Geometry: final body of the model. Coordinates: model frame, mm. A direction names the side the tool comes from. Give positions to 0.01 mm unless a question says otherwise; leave off trailing zeros. Loops run counter-clockwise (first coordinate to the right, second up) from the corner with the lowest first, then second, coordinate; pieces in that order, holes last.
1. First-contact query: P1, Ø1.5, axis at x = -27.5, z = 3.5, coming from the -Y side. Flat tip, straight axial feed; report the tip coordinate or a pass-through.
2. Section A-A, the plane y = 13. Output: boundary loops of the cut face in (x, z), then the cut area to 3 significant figures.
3. Access query for faces 5 (the face through (-29.15, 14.93, -0.92)), 6 (the face through (0.49, -1.745, -5.361)). Directions: +Z, -Z, +X, -X, +Y, -Y. A direction counts if a zero-diameter tool reaches every point of the face in a straight line with its end or side. Return the directions, or none.
4. Section D-D, the plane y = -0.75. Output: boundary loops of the cut face in (x, z).
5. Section C-C, the plane z = -6. Output: boundary loops of the cut face in (x, y), then the cut area to 3 significant figures.
6. Material intervals for line 1 along X through (y, z) = (6.25, -1); line 2 along X through (y, z) = (18, 0); line 3 along Z through (x, y) = (26, 15), sorted ascending.
7. Draft query along X for faces 1 (the face through (-35, 8, 0)), 2 (the face through (0, 12, 7.5)), 3 (the face through (35, 8, 0)), 4 (the face through (-29.063, 4.93, -0.902)). Return one class per face: +X half, -X half, draft (parallel to the pull), parting line (faces both ways), or undercut.
from build123d import *
from OCP.BRepFilletAPI import BRepFilletAPI_MakeChamfer

# Parameters (mm, degrees)
SKETCH1_W           = 70
SKETCH1_H           = 15
SKETCH1_R           = 4.25
BOSS_EXTRUDE1_DEPTH = 20
SKETCH2_W           = 70
SKETCH2_H           = 15
BOSS_EXTRUDE2_DEPTH = 4
FILLET1_R           = 7.5
CHAMFER1_SIZE       = 10
CHAMFER1_SIZE2      = 0.174550649


with BuildPart() as part:
    # Sketch1 → Boss-Extrude1 (new body)
    with BuildSketch(Plane(origin=(0, 0, 0), x_dir=(1, 0, 0), z_dir=(0, 1, 0))):
        Rectangle(SKETCH1_W, SKETCH1_H)
        with Locations(Location((-25, 0, 0), (0, 0, 270))):
            Circle(SKETCH1_R, mode=Mode.SUBTRACT)
        with Locations(Location((25, 0, 0), (0, 0, 270))):
            Circle(SKETCH1_R, mode=Mode.SUBTRACT)
    extrude(amount=BOSS_EXTRUDE1_DEPTH)

    # Sketch2 → Boss-Extrude2 (add)
    with BuildSketch(Plane.XZ):
        Rectangle(SKETCH2_W, SKETCH2_H)
    extrude(amount=BOSS_EXTRUDE2_DEPTH)

    # Fillet1
    fillet1_edges = [part.edges().sort_by_distance(p)[0] for p in [
        (0, -4, 7.5),
        (0, -4, -7.5),
    ]]
    fillet(fillet1_edges, radius=FILLET1_R - 0.0001)  # a hair under: the kernel refuses the full size

    # Chamfer1: one chamfer whose edges measure the first distance from different faces: ONE call of the kernel's chamfer builder (chamfer() names one face for all edges)
    chamfer1_edges_1 = [part.edges().sort_by_distance(p)[0] for p in [
        (-25, 0, -4.25),
    ]]
    chamfer1_side_1 = [part.faces().sort_by_distance(p)[0] for p in [
        (-25, 10, -4.25),
    ]]
    chamfer1_edges_2 = [part.edges().sort_by_distance(p)[0] for p in [
        (25, 0, -4.25),
    ]]
    chamfer1_side_2 = [part.faces().sort_by_distance(p)[0] for p in [
        (25, 10, -4.25),
    ]]
    chamfer1 = BRepFilletAPI_MakeChamfer(part.part.solid().wrapped)
    for e in chamfer1_edges_1:
        chamfer1.Add(CHAMFER1_SIZE, CHAMFER1_SIZE2, e.wrapped, chamfer1_side_1[0].wrapped)  # the first distance lies on this face
    for e in chamfer1_edges_2:
        chamfer1.Add(CHAMFER1_SIZE, CHAMFER1_SIZE2, e.wrapped, chamfer1_side_2[0].wrapped)  # the first distance lies on this face
    add(Compound.cast(chamfer1.Shape()), mode=Mode.REPLACE)


solid = part.part
Answers below:
1. P1: stops at y = -3.48
2. outline: (-35, -7.5) - (35, -7.5) - (35, 7.5) - (-35, 7.5) - close; hole circle Ø8.5 at (-25, 0); hole circle Ø8.5 at (25, 0)
2. area: 937 mm2
3. face 5: +Y
3. face 6: -Z, +X, -X, -Y
4. outline: (-35, -6.18) - (35, -6.18) - (35, 6.18) - (-35, 6.18) - close
5. outline: (-35, -1) - (35, -1) - (35, 20) - (-35, 20) - close
5. area: 1,470 mm2
6. line 1: x = -35 to -29.06, -20.94 to 20.94, 29.06 to 35
6. line 2: x = -35 to -29.25, -20.75 to 20.75, 29.25 to 35
6. line 3: z = -7.5 to -4.13, 4.13 to 7.5
7. face 1: -X half
7. face 2: draft
7. face 3: +X half
7. face 4: undercut
